from build123d import *

# Parameters (mm, degrees)
SKETCH1_R           = 111.5
SKETCH1_R_2         = 98
BOSS_EXTRUDE1_DEPTH = 3
SKETCH2_R           = 3
CUT_EXTRUDE1_DEPTH  = 4


with BuildPart() as part:
    # Sketch1 → Boss-Extrude1 (new body)
    with BuildSketch(Plane(origin=(0, 0, 0), x_dir=(1, 0, 0), z_dir=(0, 1, 0))):
        Circle(SKETCH1_R)
        Circle(SKETCH1_R_2, mode=Mode.SUBTRACT)
    extrude(amount=BOSS_EXTRUDE1_DEPTH)

    # Sketch2 → Cut-Extrude1 (cut, through all)
    with BuildSketch(Plane(origin=(0, 3, 0), x_dir=(1, 0, 0), z_dir=(0, 1, 0))):
        with Locations((0, 105)):
            Circle(SKETCH2_R)
        with Locations((105, 0)):
            Circle(SKETCH2_R)
        with Locations((0, -105)):
            Circle(SKETCH2_R)
        with Locations((-105, 0)):
            Circle(SKETCH2_R)
    extrude(amount=-CUT_EXTRUDE1_DEPTH, mode=Mode.SUBTRACT)


solid = part.part
The listing builds one solid part. Answer for the finished solid, in the listing's coordinates (mm). Coordinates: 2 decimals unless noted, no trailing zeros. Write each loop counter-clockwise with the first axis right and the second up, starting at its lowest first coordinate (ties: lowest second). Pieces come first, ordered by that corner, then holes. Notation, with made-up numbers: (42.25, -36) - (92.25, -36) arc R16 cw to (92.25, -20) - close; hole circle Ø9 at (65.5, 68). An arc over 180 degrees is marked (long way). Answer as CSV lines item,"result".
1. Find section A-A (x = 0). Give the vertices of the cut face in (y, z).
Computed values:
outline,"(0, -111.5) - (3, -111.5) - (3, -108) - (0, -108) - close; (0, -102) - (3, -102) - (3, -98) - (0, -98) - close; (0, 98) - (3, 98) - (3, 102) - (0, 102) - close; (0, 108) - (3, 108) - (3, 111.5) - (0, 111.5) - close"
2. Determine the mould class of faces 1 (the cylindrical face through (-14.52, 1.48, -110.55)), 2 (the cylindrical face through (-0.65, 1.52, -102.07)), 3 (the cylindrical face through (52.684, 1.479, -82.634)), 4 (the flat face through (99, 0, -1)) for opening direction X: +X half, -X half, draft (parallel to the pull), parting line (faces both ways), or undercut.
Computed values:
face 1,"parting line"
face 2,"undercut"
face 3,"undercut"
face 4,"draft"
3. Find section C-C (y = 1.9). Give the vertices of the cut face in (x, z), plus the area to 3 significant figures.
Computed values:
outline,"circle Ø223 at (0, 0); hole circle Ø6 at (-105, 0); hole circle Ø196 at (0, 0); hole circle Ø6 at (0, -105); hole circle Ø6 at (0, 105); hole circle Ø6 at (105, 0)"
area,"8,770 mm²"
4. Find section D-D (x = -71). Give the vertices of the cut face in (y, z).
Computed values:
outline,"(0, -85.97) - (3, -85.97) - (3, -67.55) - (0, -67.55) - close; (0, 67.55) - (3, 67.55) - (3, 85.97) - (0, 85.97) - close"
5. Find section B-B (z = 83.5). Give the vertices of the cut face in (x, y), plus the area to 3 significant figures.
Computed values:
outline,"(-73.89, 0) - (-51.3, 0) - (-51.3, 3) - (-73.89, 3) - close; (51.3, 0) - (73.89, 0) - (73.89, 3) - (51.3, 3) - close"
area,"136 mm²"
6. Straight lines are drawn through the part: line 1 (Z direction, x = 0, y = 1.2); line 2 (Z direction, x = 52, y = 0.9). For each, find the intervals that lie inside material, in ascending order. Write a range as [from, to].
Computed values:
line 1,"z = [-111.5, -108], [-102, -98], [98, 102], [108, 111.5]"
line 2,"z = [-98.63, -83.07], [83.07, 98.63]"
